from build123d import *

# Parameters (mm, degrees)
SKETCH_1_R          = 3.25
SKETCH_1_R_2        = 3.2
EXTRUDE_1_DEPTH     = 9.5
SKETCH_2_R          = 5.2
CUT_EXTRUDE_1_DEPTH = 6.5
SKETCH_3_W          = 10.4
SKETCH_3_H          = 10.4
SKETCH_3_R          = 3.25
CUT_EXTRUDE_2_DEPTH = 6.5


with BuildPart() as part:
    # 스케치1 → 보스-돌출1 (new body)
    with BuildSketch(Plane(origin=(0, 0, 0), x_dir=(1, 0, 0), z_dir=(0, 1, 0))):
        with BuildLine():
            Line((3.446699141, -53.446699141), (-21.553300859, -78.446699141))
            ThreePointArc((-21.553300859, -78.446699141), (-23.179096494, -86.620125743), (-16.25, -91.25))
            Line((-16.25, -91.25), (33.75, -91.25))
            ThreePointArc((33.75, -91.25), (40.679096494, -86.620125743), (39.053300859, -78.446699141))
            Line((39.053300859, -78.446699141), (14.053300859, -53.446699141))
            ThreePointArc((14.053300859, -53.446699141), (8.75, -51.25), (3.446699141, -53.446699141))
        make_face()
        with Locations((0, -80)):
            Circle(SKETCH_1_R, mode=Mode.SUBTRACT)
        with Locations((-16.25, -83.75)):
            Circle(SKETCH_1_R_2, mode=Mode.SUBTRACT)
        with Locations((8.75, -58.75)):
            Circle(SKETCH_1_R_2, mode=Mode.SUBTRACT)
        with Locations((33.75, -83.75)):
            Circle(SKETCH_1_R_2, mode=Mode.SUBTRACT)
    extrude(amount=EXTRUDE_1_DEPTH)

    # 스케치2 → 컷-돌출1 (cut)
    with BuildSketch(Plane(origin=(0, 9.5, 0), x_dir=(1, 0, 0), z_dir=(0, 1, 0))):
        with Locations((8.75, -58.75)):
            Circle(SKETCH_2_R)
        with Locations((33.75, -83.75)):
            Circle(SKETCH_2_R)
        with Locations((-16.25, -83.75)):
            Circle(SKETCH_2_R)
    extrude(amount=-CUT_EXTRUDE_1_DEPTH, mode=Mode.SUBTRACT)

    # 스케치3 → 컷-돌출2 (cut)
    with BuildSketch(Plane.XZ):
        with Locations((0, 80)):
            Rectangle(SKETCH_3_W, SKETCH_3_H)
        with Locations((0, 80)):
            Circle(SKETCH_3_R, mode=Mode.SUBTRACT)
    extrude(amount=-CUT_EXTRUDE_2_DEPTH, mode=Mode.SUBTRACT)


solid = part.part
Design review of the part built by this model. Coordinates are the model's own, in mm. A direction names the side the tool comes from. Give positions to 0.01 mm unless a question says otherwise; leave off trailing zeros. Order: outer loops, then holes, each group sorted by start corner. A loop starts at its lowest first (then second) coordinate and runs counter-clockwise, first axis right, second up. Notation, with made-up numbers: (30, 11) - (70, 11) arc R13 ccw to (70, 23) - close; hole circle Ø5 at (37, 51.5). An arc over 180 degrees is marked (long way). Write item = value, one per line. Start each with the question number.
Q1. To check wall thickness, follow L1, parallel to X at y = 5.75, z = 83.75; L2, parallel to X at y = 7.25, z = 83.75; L3, parallel to X at y = 1.95, z = 83.75. State the ranges of each line that lie inside material, in increasing order. Write a range as from..to.
Q2. Clearance check with flat-ended pins moving along their axes: pin 1 Ø1 at (y, z) = (7.5, 60) entering from +X; pin 2 Ø4 at (x, y) = (11.5, 6) entering from -Z; pin 3 Ø8.5 at (x, z) = (0, 80) entering from -Y. State where each tip first meets the part, or that it passes through.
Q3. Tool access review of faces 1 (the face through (-4, 6.5, 80)), 2 (the face through (6, 3, 61)), 3 (the face through (-23.225, 4.684, 86.505)): name each direction out of +Z, -Z, +X, -X, +Y, -Y from which nothing blocks a thin tool from reaching the whole face with its end or side.
Q4. We need section D-D on y = 1.25. State the section outline as (x, z) points.
Q5. We need section A-A on y = 5.75. State the section outline as (x, z) points.
Q6. We need section C-C on z = 84.5. State the section outline as (x, y) points.
Q7. We need section B-B on x = 9. State the section outline as (y, z) points.
Q8. Mouldability with a two-part tool opening along Z and no side actions: class faces 4 (the face through (8, 0, 75)), 5 (the face through (38.553, 6.296, 85.742)), 6 (the face through (8.83, 4.68, 51.25)), 7 (the face through (0, 3, 74.8)) as released by +Z, released by -Z, zero draft, split by the parting line, or undercut.
Working result:
q1.L1 = -23.75..-21.45, -11.05..-5.2, 5.2..28.55, 38.95..41.25
q1.L2 = -23.75..-21.45, -11.05..28.55, 38.95..41.25
q1.L3 = -23.75..-19.45, -13.05..-5.2, 5.2..30.55, 36.95..41.25
q2.pin_1 = 21.11
q2.pin_2 = 51.29
q2.pin_3 = 6.5
q3.face_1 = -Y
q3.face_2 = +Y
q3.face_3 = -X, +Y, -Y
q4.outline = (-21.55, 78.45) - (3.45, 53.45) arc R7.5 ccw to (14.05, 53.45) - (39.05, 78.45) arc R7.5 ccw to (33.75, 91.25) - (-16.25, 91.25) arc R7.5 ccw to start; hole circle Ø6.4 at (-16.25, 83.75); hole (-5.2, 74.8) - (5.2, 74.8) - (5.2, 85.2) - (-5.2, 85.2) - close; hole circle Ø6.4 at (8.75, 58.75); hole circle Ø6.4 at (33.75, 83.75)
q5.outline = (-21.55, 78.45) - (3.45, 53.45) arc R7.5 ccw to (14.05, 53.45) - (39.05, 78.45) arc R7.5 ccw to (33.75, 91.25) - (-16.25, 91.25) arc R7.5 ccw to start; hole circle Ø10.4 at (-16.25, 83.75); hole (-5.2, 74.8) - (5.2, 74.8) - (5.2, 85.2) - (-5.2, 85.2) - close; hole circle Ø10.4 at (8.75, 58.75); hole circle Ø10.4 at (33.75, 83.75)
q6.outline = (-23.71, 0) - (-19.36, 0) - (-19.36, 3) - (-21.4, 3) - (-21.4, 9.5) - (-23.71, 9.5) - close; (-13.14, 0) - (-5.2, 0) - (-5.2, 6.5) - (5.2, 6.5) - (5.2, 0) - (30.64, 0) - (30.64, 3) - (28.6, 3) - (28.6, 9.5) - (-11.1, 9.5) - (-11.1, 3) - (-13.14, 3) - close; (36.86, 0) - (41.21, 0) - (41.21, 9.5) - (38.9, 9.5) - (38.9, 3) - (36.86, 3) - close
q7.outline = (0, 51.25) - (9.5, 51.25) - (9.5, 53.56) - (3, 53.56) - (3, 55.56) - (0, 55.56) - close; (0, 61.94) - (3, 61.94) - (3, 63.94) - (9.5, 63.94) - (9.5, 91.25) - (0, 91.25) - close
q8.face_4 = zero draft
q8.face_5 = undercut
q8.face_6 = released by -Z
q8.face_7 = undercut
